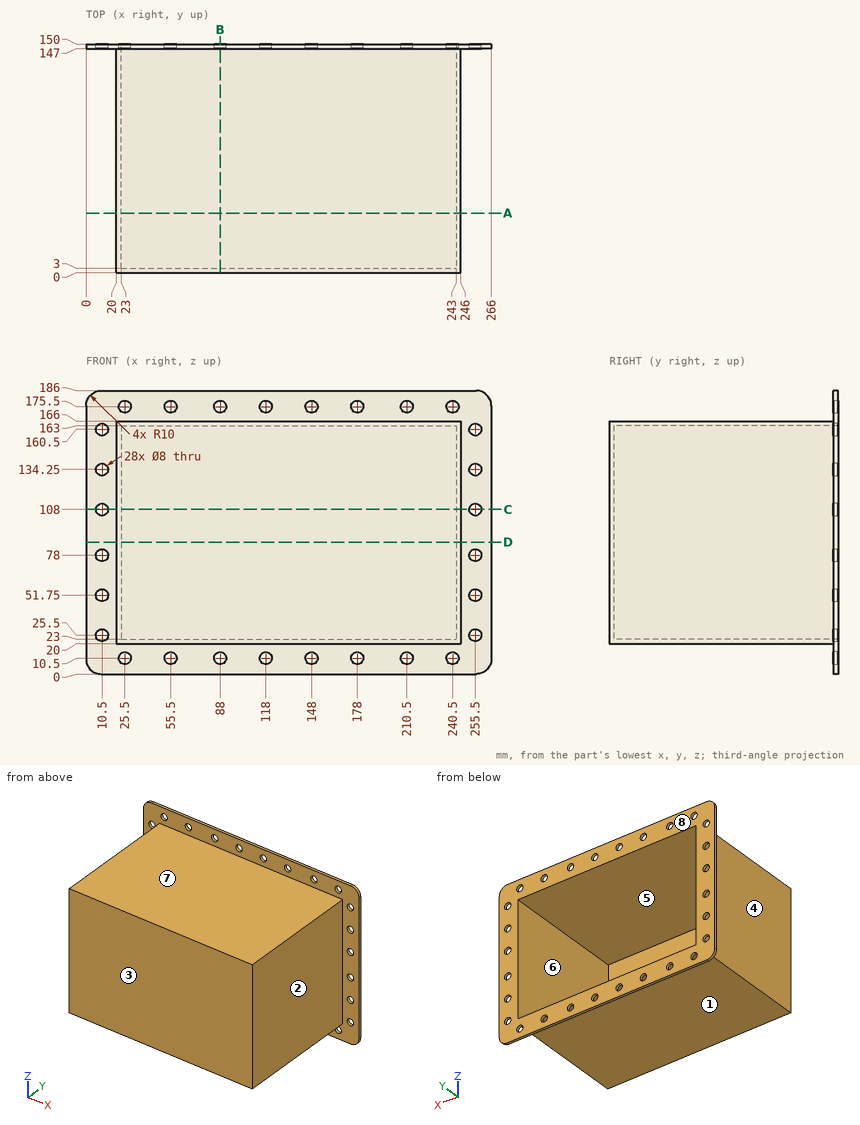
Geometry: see drawing. Coordinates: mm, zero at the bounding-box minimum. A direction names the side the tool comes from. Coordinates: 2 decimals unless noted, no trailing zeros. Loops run counter-clockwise (first coordinate to the right, second up) from the corner with the lowest first, then second, coordinate; pieces in that order, holes last. Notation, with made-up numbers: (5, 83.5) -> (9, 83.5) arc R16 cw to (9, 105.5) -> close; hole circle Ø9 at (80.25, -2). An arc over 180 degrees is marked (long way). Use a Markdown table: item, result.
1) Cut plane D-D (z = 86.5). Return the cut outline in (x, y).
Results found:
| item | result |
|---|---|
| outline | (0, 147) -> (20, 147) -> (20, 0) -> (246, 0) -> (246, 147) -> (266, 147) -> (266, 150) -> (243, 150) -> (243, 3) -> (23, 3) -> (23, 150) -> (0, 150) -> close |
2) Cut plane B-B (x = 88). Return the cut outline in (y, z), then the cut area to 3 significant figures.
Results found:
| item | result |
|---|---|
| outline | (0, 20) -> (147, 20) -> (147, 14.5) -> (150, 14.5) -> (150, 23) -> (3, 23) -> (3, 163) -> (150, 163) -> (150, 171.5) -> (147, 171.5) -> (147, 166) -> (0, 166) -> close; (147, 0) -> (150, 0) -> (150, 6.5) -> (147, 6.5) -> close; (147, 179.5) -> (150, 179.5) -> (150, 186) -> (147, 186) -> close |
| area | 1,390 mm2 |
3) Access query for the marked faces 1, 2, 3, 4 and 5. Directions: +Z, -Z, +X, -X, +Y, -Y. A direction counts if a zero-diameter tool reaches every point of the face in a straight line with its end or side. Return the directions, or none.
Results found:
| item | result |
|---|---|
| face 1 | -Z, +X, -X, -Y |
| face 2 | +Z, -Z, +X, -Y |
| face 3 | +Z, -Z, +X, -X, -Y |
| face 4 | +Z, -Z, -X, -Y |
| face 5 | +Y |
4) Cut plane A-A (y = 39). Return the cut outline in (x, z).
Results found:
| item | result |
|---|---|
| outline | (20, 20) -> (246, 20) -> (246, 166) -> (20, 166) -> close; hole (23, 23) -> (243, 23) -> (243, 163) -> (23, 163) -> close |
5) Pull-direction query (Z, two-part tool) for the marked faces 6, 7 and 8; classes: released by +Z, released by -Z, zero draft, split by the parting line, or undercut.
Results found:
| item | result |
|---|---|
| face 6 | undercut |
| face 7 | released by +Z |
| face 8 | zero draft |
6) Cut plane C-C (z = 108). Return the cut outline in (x, y).
Results found:
| item | result |
|---|---|
| outline | (0, 147) -> (6.5, 147) -> (6.5, 150) -> (0, 150) -> close; (14.5, 147) -> (20, 147) -> (20, 0) -> (246, 0) -> (246, 147) -> (251.5, 147) -> (251.5, 150) -> (243, 150) -> (243, 3) -> (23, 3) -> (23, 150) -> (14.5, 150) -> close; (259.5, 147) -> (266, 147) -> (266, 150) -> (259.5, 150) -> close |
7) Material intervals for line 1 along X through (y, z) = (147.7, 78); line 2 along X through (y, z) = (21.5, 57.5); line 3 along Z through (x, y) = (106.5, 40.5), sorted ascending. Write a range as from..to.
Results found:
| item | result |
|---|---|
| line 1 | x = 0..6.5, 14.5..23, 243..251.5, 259.5..266 |
| line 2 | x = 20..23, 243..246 |
| line 3 | z = 20..23, 163..166 |
8) Contact query for flat-ended pins moving along their axis: pin 1 (4 mm diameter, centred on y = 119, z = 52, fed in from +X); pin 2 (9 mm diameter, centred on x = 10.5, z = 134.25, fed in from -Y); pin 3 (2 mm diameter, centred on y = 120.5, z = 67, fed in from -X). Output: stop coordinate, or through.
Results found:
| item | result |
|---|---|
| pin 1 | stops at x = 246 |
| pin 2 | stops at y = 147 |
| pin 3 | stops at x = 20 |
